Here's how the part is built. I have some questions about the finished solid (model axes, mm). A direction names the side the tool comes from. Round coordinates to 2 decimals unless told otherwise and drop trailing zeros. Write each loop counter-clockwise with the first axis right and the second up, starting at its lowest first coordinate (ties: lowest second). Pieces come first, ordered by that corner, then holes. Notation, with made-up numbers: (66.5, 65.5) - (108.5, 65.5) arc R21 ccw to (108.5, 98.5) - close; hole circle Ø3 at (27.25, 87). An arc over 180 degrees is marked (long way). Write item = value, one per line. Start each with the question number.
Item 1: If I drill on line 1 along X through (y, z) = (8, -15); line 2 along Y through (x, z) = (-6.5, 37); line 3 along Z through (x, y) = (15, 14), over which ranges is the centre line in solid material (lowest first)? Write a range as [from, to].
Item 2: If we section it at A-A (y = 22.5): Please give me the cut outline in (x, z).
Item 3: Thinking about a two-plate mould opening in Z: for faces 1 (the face through (25, 34, 36)), 2 (the face through (-17, 10, 16)), 3 (the face through (0, 10, 30)), 4 (the face through (0, 20, 0)), which applies, pulls with the +Z half, pulls with the -Z half, needs draft (parallel to the pull), parting line crosses it, or undercut?
Item 4: If we section it at C-C (x = 2.5): Please give me the cut outline in (y, z), and give its area (3 significant figures).
Item 5: If we section it at B-B (x = -15): Please give me the cut outline in (y, z).
Item 6: If we section it at D-D (y = 40): Please give me the cut outline in (x, z), and give its area (3 significant figures).
Item 7: Which directions (+Z, -Z, +X, -X, +Y, -Y) give clear straight access to the entire face, cutting with the end or side of a thin tool? Please do faces 5 (the face through (15, 52, 19)), 6 (the face through (0, 22, 15)), 7 (the face through (0, 20, 36)).
Item 8: For P1, Ø6.5, axis at x = 15, z = 15, coming from the +Y side; P2, Ø4, axis at y = 35.5, z = 36.5, coming from the -X side; P3, Ø12, axis at x = -3, y = 55.5, coming from the +Z side, each with a flat end and sliding along its axis, tell me the tip position at first contact or that it passes through.
```python
from build123d import *

# Parameters (mm, degrees)
SKETCH1_W           = 60
SKETCH1_H           = 60
SKETCH1_R           = 2
BOSS_EXTRUDE1_DEPTH = 60
SKETCH2_R           = 4
CUT_EXTRUDE1_DEPTH  = 50
FILLET1_R           = 5
SKETCH3_W           = 30
SKETCH3_H           = 40
CUT_EXTRUDE2_DEPTH  = 61
SKETCH4_W           = 40
SKETCH4_H           = 19
CUT_EXTRUDE3_DEPTH  = 30
SKETCH5_W           = 50
SKETCH5_H           = 29
SKETCH5_W_2         = 40
SKETCH5_H_2         = 19
BOSS_EXTRUDE3_DEPTH = 13
SKETCH6_R           = 10
CUT_EXTRUDE4_DEPTH  = 10


with BuildPart() as part:
    # Sketch1 → Boss-Extrude1 (new body)
    with BuildSketch(Plane(origin=(0, 0, 0), x_dir=(1, 0, 0), z_dir=(0, 1, 0))):
        Rectangle(SKETCH1_W, SKETCH1_H)
        with Locations((-15, 15)):
            Circle(SKETCH1_R, mode=Mode.SUBTRACT)
        with Locations((15, 15)):
            Circle(SKETCH1_R, mode=Mode.SUBTRACT)
        with Locations((15, -15)):
            Circle(SKETCH1_R, mode=Mode.SUBTRACT)
        with Locations((-15, -15)):
            Circle(SKETCH1_R, mode=Mode.SUBTRACT)
    extrude(amount=BOSS_EXTRUDE1_DEPTH)

    # Sketch2 → Cut-Extrude1 (cut)
    with BuildSketch(Plane(origin=(0, 60, 0), x_dir=(1, 0, 0), z_dir=(0, 1, 0))):
        with Locations((-15, 15)):
            Circle(SKETCH2_R)
        with Locations((15, 15)):
            Circle(SKETCH2_R)
        with Locations((15, -15)):
            Circle(SKETCH2_R)
        with Locations((-15, -15)):
            Circle(SKETCH2_R)
    extrude(amount=-CUT_EXTRUDE1_DEPTH, mode=Mode.SUBTRACT)

    # Fillet1
    fillet1_edges = [part.edges().sort_by_distance(p)[0] for p in [
        (30, 30, 30),
        (-30, 30, 30),
        (-30, 30, -30),
        (30, 30, -30),
    ]]
    fillet(fillet1_edges, radius=FILLET1_R)

    # Sketch3 → Cut-Extrude2 (cut, through all)
    with BuildSketch(Plane(origin=(30, 0, 0), x_dir=(0, 0, -1), z_dir=(1, 0, 0))):
        with Locations((0, 40)):
            Rectangle(SKETCH3_W, SKETCH3_H)
    extrude(amount=-CUT_EXTRUDE2_DEPTH, mode=Mode.SUBTRACT)

    # Sketch4 → Cut-Extrude3 (cut)
    with BuildSketch(Plane.XY.offset(30)):
        with Locations((0, 34.5)):
            Rectangle(SKETCH4_W, SKETCH4_H)
    extrude(amount=-CUT_EXTRUDE3_DEPTH, mode=Mode.SUBTRACT)

    # Sketch5 → Boss-Extrude3 (add)
    with BuildSketch(Plane.XY.offset(30)):
        with Locations((0, 34.5)):
            Rectangle(SKETCH5_W, SKETCH5_H)
        with Locations((0, 34.5)):
            Rectangle(SKETCH5_W_2, SKETCH5_H_2, mode=Mode.SUBTRACT)
    extrude(amount=BOSS_EXTRUDE3_DEPTH)

    # Sketch6 → Cut-Extrude4 (cut)
    with BuildSketch(Plane(origin=(0, 0, -30), x_dir=(-1, 0, 0), z_dir=(0, 0, -1))):
        with Locations((0, 40)):
            Circle(SKETCH6_R)
    extrude(amount=-CUT_EXTRUDE4_DEPTH, mode=Mode.SUBTRACT)


solid = part.part
```
Reply:
q1.line_1 = [-30, -17], [-13, 13], [17, 30]
q1.line_2 = [20, 25], [44, 49]
q1.line_3 = [-30, -19], [-11, 11], [19, 30]
q2.outline = (-30, -25) arc R5 ccw to (-25, -30) - (25, -30) arc R5 ccw to (30, -25) - (30, -15) - (19, -15) arc R4 cw to (11, -15) - (-11, -15) arc R4 cw to (-19, -15) - (-30, -15) - close; (-30, 15) - (-19, 15) arc R4 cw to (-11, 15) - (11, 15) arc R4 cw to (19, 15) - (30, 15) - (30, 25) arc R5 ccw to (25, 30) - (25, 43) - (-25, 43) - (-25, 30) arc R5 ccw to (-30, 25) - close
q3.face_1 = needs draft
q3.face_2 = undercut
q3.face_3 = pulls with the +Z half
q3.face_4 = undercut
q4.outline = (0, -30) - (30.32, -30) - (30.32, -20) - (49.68, -20) - (49.68, -30) - (60, -30) - (60, -15) - (20, -15) - (20, 15) - (25, 15) - (25, 43) - (20, 43) - (20, 30) - (0, 30) - close; (44, 15) - (60, 15) - (60, 30) - (49, 30) - (49, 43) - (44, 43) - close
q4.area = 2,050 mm2
q5.outline = (0, -30) - (60, -30) - (60, -19) - (10, -19) - (10, -17) - (0, -17) - close; (0, -13) - (10, -13) - (10, -11) - (20, -11) - (20, 11) - (10, 11) - (10, 13) - (0, 13) - close; (0, 17) - (10, 17) - (10, 19) - (25, 19) - (25, 43) - (20, 43) - (20, 30) - (0, 30) - close; (44, 19) - (60, 19) - (60, 30) - (49, 30) - (49, 43) - (44, 43) - close
q6.outline = (-30, -25) arc R5 ccw to (-25, -30) - (-10, -30) - (-10, -20) - (10, -20) - (10, -30) - (25, -30) arc R5 ccw to (30, -25) - (30, -15) - (19, -15) arc R4 cw to (11, -15) - (-11, -15) arc R4 cw to (-19, -15) - (-30, -15) - close; (-30, 15) - (-20, 15) - (-20, 43) - (-25, 43) - (-25, 30) arc R5 ccw to (-30, 25) - close; (20, 15) - (30, 15) - (30, 25) arc R5 ccw to (25, 30) - (25, 43) - (20, 43) - close
q6.area = 1,060 mm2
q7.face_5 = +Y
q7.face_6 = +X, -X, +Y
q7.face_7 = +Z, +X, -X, -Y
q8.P1 = 10
q8.P2 = -25
q8.P3 = 30
